```python
from build123d import *

# Parameters (mm, degrees)
SKETCH1_R                     = 3.6195
SKETCH1_R_2                   = 4.7625
SKETCH1_R_3                   = 1.6999966
BOSS_EXTRUDE1_DEPTH           = 6.35
TAP_DRILL_FOR_6_32_TAP4_D     = 2.7051
TAP_DRILL_FOR_6_32_TAP4_DEPTH = 10.16
TAP_DRILL_FOR_6_32_TAP4_TIP   = 0.81269403
TAP_DRILL_FOR_6_32_TAP3_D     = 2.7051
TAP_DRILL_FOR_6_32_TAP3_DEPTH = 10.16
TAP_DRILL_FOR_6_32_TAP3_TIP   = 0.81269403
SKETCH11_W                    = 6.35
SKETCH11_H                    = 6.1722
BOSS_EXTRUDE2_DEPTH           = 1.016
SKETCH12_W                    = 6.35
SKETCH12_H                    = 6.1722
BOSS_EXTRUDE3_DEPTH           = 1.016
TAP_DRILL_FOR_6_32_TAP1_D     = 2.7051
TAP_DRILL_FOR_6_32_TAP1_DEPTH = 7.62
TAP_DRILL_FOR_6_32_TAP1_TIP   = 0.81269403
TAP_DRILL_FOR_6_32_TAP2_D     = 2.7051
TAP_DRILL_FOR_6_32_TAP2_DEPTH = 7.62
TAP_DRILL_FOR_6_32_TAP2_TIP   = 0.81269403
CUT_EXTRUDE1_DEPTH            = 130.67066939


with BuildPart() as part:
    # Sketch1 → Boss-Extrude1 (new body)
    with BuildSketch(Plane(origin=(0, 0, 0), x_dir=(0, 0, -1), z_dir=(1, 0, 0))):
        Polygon((0, 0), (-14.664696837, 25.4), (-112.335303163, 25.4), (-127, 0), align=None)
        with Locations((-98.298, 12.7)):
            Circle(SKETCH1_R, mode=Mode.SUBTRACT)
        with Locations((-28.702, 12.7)):
            Circle(SKETCH1_R_2, mode=Mode.SUBTRACT)
        with Locations((-89.7979916, 12.7)):
            Circle(SKETCH1_R_3, mode=Mode.SUBTRACT)
        with Locations((-106.7980084, 12.7)):
            Circle(SKETCH1_R_3, mode=Mode.SUBTRACT)
    extrude(amount=BOSS_EXTRUDE1_DEPTH)

    # Tap Drill for #6-32 Tap4
    with Locations(Plane(origin=(0, 25.4, 0), x_dir=(1, 0, 0), z_dir=(0, 1, 0))):
        with Locations((3.175, -93.285303163), (3.175, -34.984696837)):
            Hole(TAP_DRILL_FOR_6_32_TAP4_D / 2, depth=TAP_DRILL_FOR_6_32_TAP4_DEPTH)
            with Locations((0, 0, -(TAP_DRILL_FOR_6_32_TAP4_DEPTH + TAP_DRILL_FOR_6_32_TAP4_TIP / 2))):  # 118° drill point
                Cone(0, TAP_DRILL_FOR_6_32_TAP4_D / 2, TAP_DRILL_FOR_6_32_TAP4_TIP, mode=Mode.SUBTRACT)

    # Tap Drill for #6-32 Tap3
    with Locations(Plane(origin=(0, 0, 0), x_dir=(-1, 0, 0), z_dir=(0, -1, 0))):
        with Locations((-3.175, -92.71), (-3.175, -22.86)):
            Hole(TAP_DRILL_FOR_6_32_TAP3_D / 2, depth=TAP_DRILL_FOR_6_32_TAP3_DEPTH)
            with Locations((0, 0, -(TAP_DRILL_FOR_6_32_TAP3_DEPTH + TAP_DRILL_FOR_6_32_TAP3_TIP / 2))):  # 118° drill point
                Cone(0, TAP_DRILL_FOR_6_32_TAP3_D / 2, TAP_DRILL_FOR_6_32_TAP3_TIP, mode=Mode.SUBTRACT)

    # Sketch11 → Boss-Extrude2 (add)
    with BuildSketch(Plane(origin=(0, 54.99261314, 95.25), x_dir=(1, 0, 0), z_dir=(0, 0.5000000000000038, 0.8660254037844366))):
        with Locations((3.175, -54.0639)):
            Rectangle(SKETCH11_W, SKETCH11_H)
    extrude(amount=BOSS_EXTRUDE2_DEPTH)

    # Sketch12 → Boss-Extrude3 (add)
    with BuildSketch(Plane(origin=(0, 0, 0), x_dir=(-1, 0, 0), z_dir=(0, 0.499999999999998, -0.8660254037844397))):
        with Locations((-3.175, 9.4361)):
            Rectangle(SKETCH12_W, SKETCH12_H)
    extrude(amount=BOSS_EXTRUDE3_DEPTH)

    # Tap Drill for #6-32 Tap1
    with Locations(Plane(origin=(0, 54.99261314, 95.25), x_dir=(1, 0, 0), z_dir=(0, 0.5000000000000038, 0.8660254037844366))):
        with Locations((3.175, -44.330606325)):
            Hole(TAP_DRILL_FOR_6_32_TAP1_D / 2, depth=TAP_DRILL_FOR_6_32_TAP1_DEPTH)
            with Locations((0, 0, -(TAP_DRILL_FOR_6_32_TAP1_DEPTH + TAP_DRILL_FOR_6_32_TAP1_TIP / 2))):  # 118° drill point
                Cone(0, TAP_DRILL_FOR_6_32_TAP1_D / 2, TAP_DRILL_FOR_6_32_TAP1_TIP, mode=Mode.SUBTRACT)

    # Tap Drill for #6-32 Tap2
    with Locations(Plane(origin=(0, 0, 0), x_dir=(-1, 0, 0), z_dir=(0, 0.499999999999998, -0.8660254037844397))):
        with Locations((-3.175, 19.169393675)):
            Hole(TAP_DRILL_FOR_6_32_TAP2_D / 2, depth=TAP_DRILL_FOR_6_32_TAP2_DEPTH)
            with Locations((0, 0, -(TAP_DRILL_FOR_6_32_TAP2_DEPTH + TAP_DRILL_FOR_6_32_TAP2_TIP / 2))):  # 118° drill point
                Cone(0, TAP_DRILL_FOR_6_32_TAP2_D / 2, TAP_DRILL_FOR_6_32_TAP2_TIP, mode=Mode.SUBTRACT)

    # Sketch19 → Cut-Extrude1 (cut, through all)
    with BuildSketch(Plane.ZY):
        Polygon((80.96083814, 20.6375), (36.6395, 20.6375), (36.6395, 6.099080191), align=None)
        Polygon((85.0354916, 4.7625), (85.0354916, 19.300919809), (40.71415346, 4.7625), align=None)
        Polygon((20.7645, 20.6375), (20.7645, 4.7625), (10.081979076, 4.7625), (19.247414599, 20.6375), align=None)
    extrude(amount=-CUT_EXTRUDE1_DEPTH, mode=Mode.SUBTRACT)


solid = part.part
```
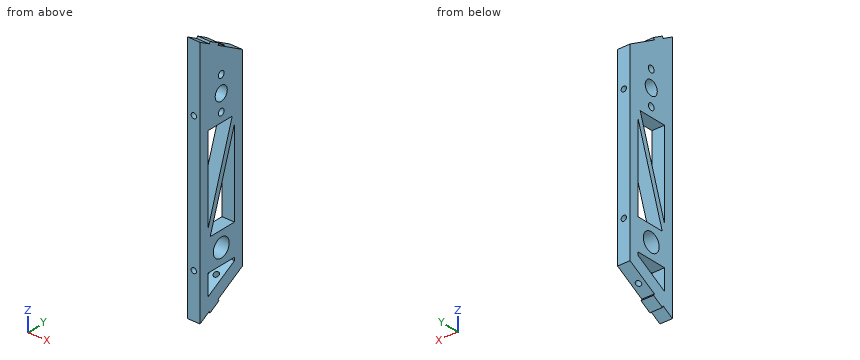
The model under review builds one solid part; all positions refer to its coordinate system, in mm. Give positions to 0.01 mm unless a question says otherwise; leave off trailing zeros. Order: outer loops, then holes, each group sorted by start corner. A loop starts at its lowest first (then second) coordinate and runs counter-clockwise, first axis right, second up. Notation, with made-up numbers: (76, 6.25) - (120, 6.25) arc R26 cw to (120, 23.25) - close; hole circle Ø10 at (9.25, 75.25). An arc over 180 degrees is marked (long way). Use CSV: the item, a comma, the result in double quotes. Start each with the question number.
Q1. We need section B-B, the plane y = 22.5. Write out the cut boundary in (x, z) (3 decimals), and give its area (3 significant figures).
Q2. To check wall thickness, follow line 1 along X through (y, z) = (2.75, 92.71); line 2 along Y through (x, z) = (2.75, 64.5); line 3 along Y through (x, z) = (2.25, 70.5). State the ranges of each line that lie inside material, in increasing order. Write a range as [from, to].
Q3. We need section C-C, the plane y = 2. Write out the cut boundary in (x, z) (3 decimals), and give its area (3 significant figures).
Q4. Clearance check with flat-ended pins moving along their axes: pin 1 Ø7.5 at (y, z) = (12.7, 28.702) entering from +X; pin 2 Ø1.9 at (x, y) = (3.5, 9.5) entering from -Z; pin 3 Ø3 at (x, y) = (2, 14.5) entering from +Z. State where each tip first meets the part, or that it passes through.
Q5. We need section A-A, the plane z = 77. Write out the cut boundary in (x, y), and give its area (3 significant figures).
Outcome:
1,outline,"(0, 12.99) - (6.35, 12.99) - (6.35, 114.01) - (0, 114.01) - close; hole circle Ø2.705 at (3.175, 34.985); hole circle Ø2.705 at (3.175, 93.285)"
1,area,"630 mm^2"
2,line 1,"x = [0, 1.82], [4.53, 6.35]"
2,line 2,"y = [0, 4.76], [12.56, 15.24], [20.64, 25.4]"
2,line 3,"y = [0, 4.76], [14.53, 17.21], [20.64, 25.4]"
3,outline,"(0, 1.155) - (6.35, 1.155) - (6.35, 125.845) - (0, 125.845) - close; hole circle Ø2.705 at (3.175, 22.86); hole circle Ø2.705 at (3.175, 92.71)"
3,area,"780 mm^2"
4,pin 1,"passes through"
4,pin 2,"stops at z = 3.76"
4,pin 3,"stops at z = 119.49"
5,outline,"(0, 0) - (6.35, 0) - (6.35, 4.76) - (0, 4.76) - close; (0, 16.67) - (6.35, 16.67) - (6.35, 19.34) - (0, 19.34) - close; (0, 20.64) - (6.35, 20.64) - (6.35, 25.4) - (0, 25.4) - close"
5,area,"77.5 mm^2"
